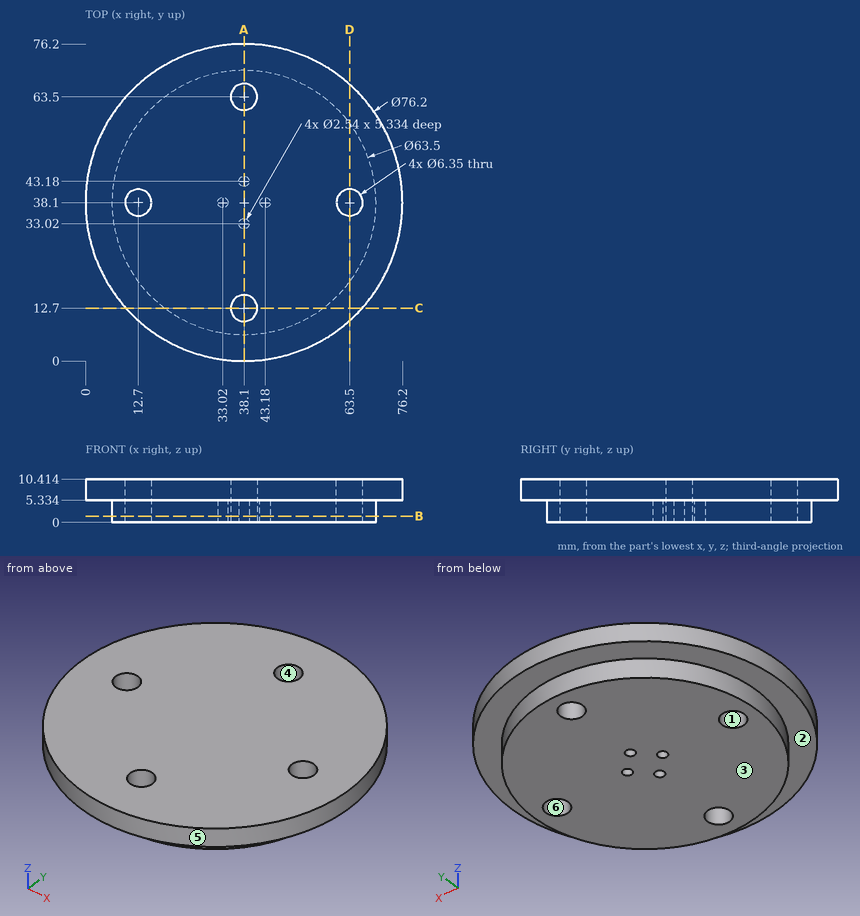
Input: dimensioned drawing with shaded views. Units: mm. Origin: part minimum x, y, z. A direction names the side the tool comes from. Give positions to 0.01 mm unless a question says otherwise; leave off trailing zeros. Order: outer loops, then holes, each group sorted by start corner. A loop starts at its lowest first (then second) coordinate and runs counter-clockwise, first axis right, second up.
(1) Section query B-B (z = 1.5). State how many separate pieces and enclosed holes the cut face has, plus the area to 3 significant figures.
(2) Pull-direction query (Y, two-part tool) for the marked faces 3, 4, 5 and 6; classes: +Y half, -Y half, draft (parallel to the pull), parting line (faces both ways), or undercut.
(3) Section query A-A (x = 38.1). Return the cut outline in (y, z) (3 decimals), plus the area to 3 significant figures.
(4) Access query for the marked faces 1 and 2. Directions: +Z, -Z, +X, -X, +Y, -Y. A direction counts if a zero-diameter tool reaches every point of the face in a straight line with its end or side. Return the directions, or none.
(5) Contact query for flat-ended pins moving along their axis: P1, Ø7.5, axis at x = 38.1, y = 63.5, coming from the -Z side; P2, Ø1.3, axis at x = 43.5, y = 38.5, coming from the -Z side; P3, Ø1, axis at x = 20.5, z = 3, coming from the +Y side; P4, Ø6, axis at y = 45.5, z = 2.5, coming from the -X side. Output: stop coordinate, or through.
(6) Material intervals for line 1 along Z through (x, y) = (21.5, 70); line 2 along Y through (x, z) = (40, 7.25); line 3 along X through (y, z) = (34, 4.5), sorted ascending.
(7) Section query C-C (y = 12.7). Return the cut outline in (x, z) (3 decimals).
Outcome:
1. separate pieces: 1
1. enclosed holes: 8
1. area: 3,020 mm2
2. face 3: draft
2. face 4: undercut
2. face 5: parting line
2. face 6: undercut
3. outline: (0, 5.334) - (6.35, 5.334) - (6.35, 0) - (9.525, 0) - (9.525, 10.414) - (0, 10.414) - close; (15.875, 0) - (31.75, 0) - (31.75, 5.334) - (34.29, 5.334) - (34.29, 0) - (41.91, 0) - (41.91, 5.334) - (44.45, 5.334) - (44.45, 0) - (60.325, 0) - (60.325, 10.414) - (15.875, 10.414) - close; (66.675, 0) - (69.85, 0) - (69.85, 5.334) - (76.2, 5.334) - (76.2, 10.414) - (66.675, 10.414) - close
3. area: 566 mm2
4. face 1: +Z, -Z
4. face 2: -Z
5. P1: stops at z = 0
5. P2: stops at z = 5.33
5. P3: stops at y = 64.85
5. P4: stops at x = 0.54
6. line 1: z = 5.33 to 10.41
6. line 2: y = 0.05 to 10.16, 15.24 to 60.96, 66.04 to 76.15
6. line 3: x = 6.62 to 37.29, 38.91 to 69.58
7. outline: (9.702, 5.334) - (19.05, 5.334) - (19.05, 0) - (34.925, 0) - (34.925, 10.414) - (9.702, 10.414) - close; (41.275, 0) - (57.15, 0) - (57.15, 5.334) - (66.498, 5.334) - (66.498, 10.414) - (41.275, 10.414) - close
